Here's how the part is built. I have some questions about the finished solid (model axes, mm). Round coordinates to 2 decimals unless told otherwise and drop trailing zeros. Order: outer loops, then holes, each group sorted by start corner. A loop starts at its lowest first (then second) coordinate and runs counter-clockwise, first axis right, second up. Notation, with made-up numbers: M -7.75,24 L 33.25,24 A12 cw 33.25,39 Z; hole C 10,75 d2. An arc over 180 degrees is marked long. Write item = value, one per line. Start each with the question number.
Item 1: I want a section at A-A, the plane z = 1.75. List the corners of the cut face in (x, y) for me.
Item 2: I want a section at D-D, the plane z = 14.5. List the corners of the cut face in (x, y) for me, plus the area to 3 significant figures.
Item 3: I want a section at C-C, the plane x = -0.25. State how many separate pieces and enclosed holes the cut face has, plus the area to 3 significant figures.
Item 4: I want a section at B-B, the plane z = 9.75. List the corners of the cut face in (x, y) for me, plus the area to 3 significant figures.
Item 5: Please list where these lines run through material, in increasing order: L1, parallel to Y at x = -0.25, z = 4.75; L2, parallel to X at y = 0, z = 10; L3, parallel to Y at x = 0, z = 15.
Item 6: I'm going to push flat-ended pins straight in: P1, Ø5.5, axis at x = 0.5, y = 0, coming from the +Z side; P2, Ø3, axis at y = 0.5, z = 3.5, coming from the -X side; P3, Ø1, axis at x = -3.5, y = 2, coming from the -Z side; P4, Ø5, axis at x = -3, z = 12, coming from the +Y side. Where does each tip first touch, or does it pass through?
Item 7: We'd pull the mould along Z, two halves only. Please class faces 1 (the face through (2, -2, 12.5)), 2 (the face through (3.142, 2.522, 7.355)), 3 (the face through (-0.11, 3.61, 3.49)): pulls with the +Z half, pulls with the -Z half, needs draft (parallel to the pull), parting line crosses it, or undercut.
```python
from build123d import *

# Parameters (mm, degrees)
ESQUISSE1_R             = 4.75
BOSS_EXTRU_1_DEPTH      = 16.8
ESQUISSE2_R             = 3.5
ENL_V_MAT_EXTRU_1_DEPTH = 4.3
ESQUISSE3_R             = 2.5
ENL_V_MAT_EXTRU_2_DEPTH = 15.190665946
ENL_V_MAT_EXTRU_3_DEPTH = 20.883036391
ENL_V_MAT_EXTRU_4_DEPTH = 20.883036548
ESQUISSE6_R             = 1
ENL_V_MAT_EXTRU_5_DEPTH = 20.883036548


with BuildPart() as part:
    # Esquisse1 → Boss.-Extru.1 (new body)
    with BuildSketch(Plane.XY):
        Circle(ESQUISSE1_R)
    extrude(amount=BOSS_EXTRU_1_DEPTH)

    # Esquisse2 → Enlèv. mat.-Extru.1 (cut)
    with BuildSketch(Plane.XY.offset(16.8)):
        Circle(ESQUISSE2_R)
    extrude(amount=-ENL_V_MAT_EXTRU_1_DEPTH, mode=Mode.SUBTRACT)

    # Esquisse3 → Enlèv. mat.-Extru.2 (cut, through all)
    with BuildSketch(Plane.XY.offset(12.5)):
        Circle(ESQUISSE3_R)
    extrude(amount=-ENL_V_MAT_EXTRU_2_DEPTH, mode=Mode.SUBTRACT)

    # Esquisse4 → Enlèv. mat.-Extru.3 (cut, through all)
    with BuildSketch(Plane(origin=(-4.749906239, 0.029844934, 0), x_dir=(0, 0, 1), z_dir=(-0.9999802608561372, 0.006283143965558955, 0))):
        with BuildLine():
            Line((0, 2.5), (5.7, 2.5))
            ThreePointArc((5.7, 2.5), (8.2, 0), (5.7, -2.5))
            Line((5.7, -2.5), (0, -2.5))
            Line((0, -2.5), (0, 2.5))
        make_face()
    extrude(amount=-ENL_V_MAT_EXTRU_3_DEPTH, mode=Mode.SUBTRACT)

    # Esquisse5 → Enlèv. mat.-Extru.4 (cut, through all)
    with BuildSketch(Plane(origin=(-0.029844934, -4.749906239, 0), x_dir=(0.9999802608561372, -0.006283143965558958, 0), z_dir=(-0.006283143965558958, -0.9999802608561372, 0))):
        with BuildLine():
            Line((5, 8.2), (8.5, 8.2))
            Line((8.5, 8.2), (8.5, -0.8))
            Line((8.5, -0.8), (-6.868883302, -0.8))
            Line((-6.868883302, -0.8), (-6.868883302, 8.2))
            Line((-6.868883302, 8.2), (-5, 8.2))
            ThreePointArc((-5, 8.2), (-3.232233047, 7.467766953), (-2.5, 5.7))
            Line((-2.5, 5.7), (-2.5, 2.5))
            ThreePointArc((-2.5, 2.5), (0, 0), (2.5, 2.5))
            Line((2.5, 2.5), (2.5, 5.7))
            ThreePointArc((2.5, 5.7), (3.232233047, 7.467766953), (5, 8.2))
        make_face()
    extrude(amount=-ENL_V_MAT_EXTRU_4_DEPTH, mode=Mode.SUBTRACT)

    # Esquisse6 → Enlèv. mat.-Extru.5 (cut, through all)
    with BuildSketch(Plane(origin=(-0.029844934, -4.749906239, 0), x_dir=(0.9999802608561372, -0.006283143965558958, 0), z_dir=(-0.006283143965558958, -0.9999802608561372, 0))):
        with Locations((0, 2.5)):
            Circle(ESQUISSE6_R)
    extrude(amount=-ENL_V_MAT_EXTRU_5_DEPTH, mode=Mode.SUBTRACT)


solid = part.part
```
Filled in:
q1.outline = M -2.41,-4.09 A4.75 ccw -0.69,-4.7 L -0.68,-2.5 L -2.4,-2.48 Z; M -2.37,2.51 L -0.65,2.5 L -0.63,4.71 A4.75 ccw -2.36,4.12 Z; M 0.63,-4.71 A4.75 ccw 2.36,-4.12 L 2.37,-2.51 L 0.65,-2.5 Z; M 0.68,2.5 L 2.4,2.48 L 2.41,4.09 A4.75 ccw 0.69,4.7 Z
q2.outline = C 0,0 d9.5; hole C 0,0 d7
q2.area = 32.4 mm^2
q3.separate_pieces = 4
q3.enclosed_holes = 0
q3.area = 58.3 mm^2
q4.outline = C 0,0 d9.5; hole C 0,0 d5
q4.area = 51.2 mm^2
q5.L1 = -4.74 to -2.5, 2.5 to 4.74
q5.L2 = -4.75 to -2.5, 2.5 to 4.75
q5.L3 = -4.75 to -3.5, 3.5 to 4.75
q6.P1 = 12.5
q6.P2 = through
q6.P3 = 7.22
q6.P4 = 4.72
q7.face_1 = pulls with the +Z half
q7.face_2 = pulls with the -Z half
q7.face_3 = undercut
